```python
from build123d import *

# Parameters (mm, degrees)
SKETCH_1_R      = 1.5
EXTRUDE_1_DEPTH = 2


with BuildPart() as part:
    # 草图1 → 凸台-拉伸1 (new body)
    with BuildSketch(Plane(origin=(0, 0, 0), x_dir=(1, 0, 0), z_dir=(0, 1, 0))):
        with BuildLine():
            Line((-65.5, 10), (-62.5, 10))
            ThreePointArc((-62.5, 10), (-52.5, 0), (-62.5, -10))
            Line((-62.5, -10), (-65.5, -10))
            ThreePointArc((-65.5, -10), (-66.914213562, -10.585786438), (-67.5, -12))
            Line((-67.5, -12), (-67.5, -50))
            ThreePointArc((-67.5, -50), (-64.571067812, -57.071067812), (-57.5, -60))
            Line((-57.5, -60), (57.5, -60))
            ThreePointArc((57.5, -60), (64.571067812, -57.071067812), (67.5, -50))
            Line((67.5, -50), (67.5, -12))
            ThreePointArc((67.5, -12), (66.914213562, -10.585786438), (65.5, -10))
            Line((65.5, -10), (62.5, -10))
            ThreePointArc((62.5, -10), (52.5, 0), (62.5, 10))
            Line((62.5, 10), (65.5, 10))
            ThreePointArc((65.5, 10), (66.914213562, 10.585786438), (67.5, 12))
            Line((67.5, 12), (67.5, 50))
            ThreePointArc((67.5, 50), (64.571067812, 57.071067812), (57.5, 60))
            Line((57.5, 60), (-57.5, 60))
            ThreePointArc((-57.5, 60), (-64.571067812, 57.071067812), (-67.5, 50))
            Line((-67.5, 50), (-67.5, 12))
            ThreePointArc((-67.5, 12), (-66.914213562, 10.585786438), (-65.5, 10))
        make_face()
        with Locations(Location((-64.5, 30, 0), (0, 0, 270))):
            Circle(SKETCH_1_R, mode=Mode.SUBTRACT)
        with Locations(Location((64.5, 30, 0), (0, 0, 270))):
            Circle(SKETCH_1_R, mode=Mode.SUBTRACT)
        with Locations(Location((64.5, -30, 0), (0, 0, 270))):
            Circle(SKETCH_1_R, mode=Mode.SUBTRACT)
        with Locations(Location((-64.5, -30, 0), (0, 0, 270))):
            Circle(SKETCH_1_R, mode=Mode.SUBTRACT)
        with Locations(Location((-64.5, 22, 0), (0, 0, 270))):
            Circle(SKETCH_1_R, mode=Mode.SUBTRACT)
        with Locations(Location((64.5, 22, 0), (0, 0, 90))):
            Circle(SKETCH_1_R, mode=Mode.SUBTRACT)
        with Locations(Location((64.5, -22, 0), (0, 0, 270))):
            Circle(SKETCH_1_R, mode=Mode.SUBTRACT)
        with Locations(Location((-64.5, -22, 0), (0, 0, 90))):
            Circle(SKETCH_1_R, mode=Mode.SUBTRACT)
    extrude(amount=EXTRUDE_1_DEPTH)


solid = part.part
```
The model under review builds one solid part; all positions refer to its coordinate system, in mm. Round coordinates to 2 decimals unless told otherwise and drop trailing zeros. Order: outer loops, then holes, each group sorted by start corner. A loop starts at its lowest first (then second) coordinate and runs counter-clockwise, first axis right, second up.
Item 1: Add section A-A, the plane z = 22. State the section outline as (x, y) points, and give its area (3 significant figures).
Working result:
outline: (-67.5, 0) - (-66, 0) - (-66, 2) - (-67.5, 2) - close; (-63, 0) - (63, 0) - (63, 2) - (-63, 2) - close; (66, 0) - (67.5, 0) - (67.5, 2) - (66, 2) - close
area: 258 mm2
Item 2: For pin 1 (1 mm diameter, centred on x = 64, y = 0.5, fed in from -Z); pin 2 (0.6 mm diameter, centred on x = 64.5, y = 1, fed in from +Z); pin 3 (1 mm diameter, centred on x = -64, y = 0.5, fed in from +Z), all flat-tipped, find the tip position at first contact; note any pin that passes through.
Working result:
pin 1: stops at z = -58
pin 2: stops at z = 57.42
pin 3: stops at z = 58
Item 3: Draft analysis for pull direction X (two halves, no side actions). For faces 1 (the cylindrical face through (-64.49, 0.99, -57.15)), 2 (the cylindrical face through (63, 1, -22)), 3 (the flat face through (-1, 2, -1)), state which applies: released by +X, released by -X, zero draft, split by the parting line, or undercut.
Working result:
face 1: released by -X
face 2: undercut
face 3: zero draft
Item 4: Add section B-B, the plane y = 1.35. Count the separate pieces of the cut face and the enclosed holes in it, and give its area (3 significant figures).
Working result:
separate pieces: 1
enclosed holes: 8
area: 15,500 mm2
Item 5: Add section C-C, the plane z = 0. State the section outline as (x, y) points.
Working result:
outline: (-52.5, 0) - (52.5, 0) - (52.5, 2) - (-52.5, 2) - close
Item 6: To check wall thickness, follow probe 1 along X at (y, z) = (1, -22); probe 2 along Z at (x, y) = (-64.5, 1.25); probe 3 along Z at (x, y) = (-54, 0.55). State the ranges of each line that lie inside material, in increasing order.
Working result:
probe 1: x = -67.5 to -66, -63 to 63, 66 to 67.5
probe 2: z = -57.14 to -31.5, -28.5 to -23.5, -20.5 to -10, 10 to 20.5, 23.5 to 28.5, 31.5 to 57.14
probe 3: z = -60 to -5.27, 5.27 to 60
